Source: CAD feature listing. Evaluate the final solid. Frame: model axes, mm. A direction names the side the tool comes from. Give positions to 0.01 mm unless a question says otherwise; leave off trailing zeros. Loops run counter-clockwise (first coordinate to the right, second up) from the corner with the lowest first, then second, coordinate; pieces in that order, holes last. Notation, with made-up numbers: M 7.25,69.5 L 46.25,69.5 A34 ccw 46.25,99.5 Z; hole C 59,-11 d3. An arc over 180 degrees is marked long. Put each result on its own line as item: value. Start each with the question number.
```python
from build123d import *

# Parameters (mm, degrees)
TOP_DEPTH          = 30
PROFILE_3_W        = 96
PROFILE_3_H        = 17
SIDE_DEPTH         = 3
PROFILE_6_W        = 96
PROFILE_6_H        = 3
BEND_DEPTH         = 9
SCREWPLATE_START   = -7
PROFILE_7_R        = 2.5
PROFILE_7_R_2      = 2
SCREWPLATE_DEPTH   = 2
SIDE2_START        = -30
PROFILE_8_W        = 96
PROFILE_8_H        = 17
SIDE2_DEPTH        = 3
BEND2_START        = -30
PROFILE_9_W        = 96
PROFILE_9_H        = 3
BEND2_DEPTH        = 9
SCREWPLATE2_START  = -21
PROFILE_10_R       = 2.5
PROFILE_10_R_2     = 2
SCREWPLATE2_DEPTH  = 2
SKETCH3_R          = 2
CUT_EXTRUDE4_DEPTH = 2
CUT_EXTRUDE5_START = -1
SKETCH3_3_R        = 4
SKETCH3_3_R_2      = 2
CUT_EXTRUDE5_DEPTH = 1


with BuildPart() as part:
    # Profile → Top (new body)
    with BuildSketch(Plane.XY):
        Polygon((97.259067876, 0), (87.259067876, 0), (-32.740932124, 0), (-42.740932124, 0), (-42.740932124, 2), (97.259067876, 2), align=None)
    extrude(amount=-TOP_DEPTH)

    # Profile<3> → Side (add)
    with BuildSketch(Plane.XY):
        with Locations((27.259067876, -8.5)):
            Rectangle(PROFILE_3_W, PROFILE_3_H)
    extrude(amount=-SIDE_DEPTH)

    # Profile<6> → Bend (add)
    with BuildSketch(Plane.XY):
        with Locations((27.259067876, -18.5)):
            Rectangle(PROFILE_6_W, PROFILE_6_H)
    extrude(amount=-BEND_DEPTH)

    # Profile<7> → ScrewPlate (add)
    with BuildSketch(Plane.XY.offset(SCREWPLATE_START)):
        Polygon((75.259067876, -20), (-20.740932124, -20), (-20.740932124, -35), (7.259067876, -35), (7.259067876, -60), (27.259067876, -60), (47.259067876, -60), (47.259067876, -35), (75.259067876, -35), align=None)
        with Locations((17.259067876, -47.5)):
            Circle(PROFILE_7_R, mode=Mode.SUBTRACT)
        with Locations((37.259067876, -47.5)):
            Circle(PROFILE_7_R, mode=Mode.SUBTRACT)
        with Locations((-15.740932124, -27)):
            Circle(PROFILE_7_R_2, mode=Mode.SUBTRACT)
        with Locations((70.259067876, -27)):
            Circle(PROFILE_7_R_2, mode=Mode.SUBTRACT)
    extrude(amount=-SCREWPLATE_DEPTH)

    # Profile<8> → Side2 (add)
    with BuildSketch(Plane.XY.offset(SIDE2_START)):
        with Locations((27.259067876, -8.5)):
            Rectangle(PROFILE_8_W, PROFILE_8_H)
    extrude(amount=SIDE2_DEPTH)

    # Profile<9> → Bend2 (add)
    with BuildSketch(Plane.XY.offset(BEND2_START)):
        with Locations((27.259067876, -18.5)):
            Rectangle(PROFILE_9_W, PROFILE_9_H)
    extrude(amount=BEND2_DEPTH)

    # Profile<10> → ScrewPlate2 (add)
    with BuildSketch(Plane.XY.offset(SCREWPLATE2_START)):
        Polygon((75.259067876, -20), (-20.740932124, -20), (-20.740932124, -35), (7.259067876, -35), (7.259067876, -60), (27.259067876, -60), (47.259067876, -60), (47.259067876, -35), (75.259067876, -35), align=None)
        with Locations((17.259067876, -47.5)):
            Circle(PROFILE_10_R, mode=Mode.SUBTRACT)
        with Locations((37.259067876, -47.5)):
            Circle(PROFILE_10_R, mode=Mode.SUBTRACT)
        with Locations((-15.740932124, -27)):
            Circle(PROFILE_10_R_2, mode=Mode.SUBTRACT)
        with Locations((70.259067876, -27)):
            Circle(PROFILE_10_R_2, mode=Mode.SUBTRACT)
    extrude(amount=-SCREWPLATE2_DEPTH)

    # Sketch3 → Cut-Extrude4 (cut)
    with BuildSketch(Plane(origin=(0, 2, 0), x_dir=(1, 0, 0), z_dir=(0, 1, 0))):
        with Locations(Location((19.259067876, 20, 0), (0, 0, 270))):
            Circle(SKETCH3_R)
        with Locations(Location((35.259067876, 20, 0), (0, 0, 270))):
            Circle(SKETCH3_R)
        with Locations(Location((35.259067876, 10, 0), (0, 0, 270))):
            Circle(SKETCH3_R)
        with Locations(Location((19.259067876, 10, 0), (0, 0, 270))):
            Circle(SKETCH3_R)
    extrude(amount=-CUT_EXTRUDE4_DEPTH, mode=Mode.SUBTRACT)

    # Sketch3<3> → Cut-Extrude5 (cut)
    # profile 1 of 4: a face of its own
    with BuildSketch(Plane(origin=(0, 2, 0), x_dir=(1, 0, 0), z_dir=(0, 1, 0)).offset(CUT_EXTRUDE5_START)):
        with Locations(Location((19.259067876, 20, 0), (0, 0, 270))):
            Circle(SKETCH3_3_R)
        with Locations(Location((19.259067876, 20, 0), (0, 0, 270))):
            Circle(SKETCH3_3_R_2, mode=Mode.SUBTRACT)
    # profile 2 of 4: a face of its own
    with BuildSketch(Plane(origin=(0, 2, 0), x_dir=(1, 0, 0), z_dir=(0, 1, 0)).offset(CUT_EXTRUDE5_START)):
        with Locations(Location((35.259067876, 20, 0), (0, 0, 270))):
            Circle(SKETCH3_3_R)
        with Locations(Location((35.259067876, 20, 0), (0, 0, 270))):
            Circle(SKETCH3_3_R_2, mode=Mode.SUBTRACT)
    # profile 3 of 4: a face of its own
    with BuildSketch(Plane(origin=(0, 2, 0), x_dir=(1, 0, 0), z_dir=(0, 1, 0)).offset(CUT_EXTRUDE5_START)):
        with Locations(Location((35.259067876, 10, 0), (0, 0, 270))):
            Circle(SKETCH3_3_R)
        with Locations(Location((35.259067876, 10, 0), (0, 0, 270))):
            Circle(SKETCH3_3_R_2, mode=Mode.SUBTRACT)
    # profile 4 of 4: a face of its own
    with BuildSketch(Plane(origin=(0, 2, 0), x_dir=(1, 0, 0), z_dir=(0, 1, 0)).offset(CUT_EXTRUDE5_START)):
        with Locations(Location((19.259067876, 10, 0), (0, 0, 270))):
            Circle(SKETCH3_3_R)
        with Locations(Location((19.259067876, 10, 0), (0, 0, 270))):
            Circle(SKETCH3_3_R_2, mode=Mode.SUBTRACT)
    extrude(amount=-CUT_EXTRUDE5_DEPTH, mode=Mode.SUBTRACT)


solid = part.part
```
1. Ray query, line 1 (Z direction, x = -7, y = -3.5); line 2 (Z direction, x = 37, y = -35); line 3 (Y direction, x = -10.5, z = -21.75). Return the intervals inside material, ascending.
2. Section D-D, the plane z = -19.75. Output: boundary loops of the cut face in (x, y).
3. Section C-C, the plane x = 28.5. Output: boundary loops of the cut face in (y, z).
4. Pull-direction query (Y, two-part tool) for faces 1 (the face through (27, -20, -3)), 2 (the face through (34, 1, -12)), 3 (the face through (33.485, 1.507, -9.077)); classes: released by +Y, released by -Y, zero draft, split by the parting line, or undercut.
5. Set-up query: faces 4 (the face through (34, 1, -22)), 5 (the face through (21.242, 1.507, -20.26)), 6 (the face through (27, -17, -24)). Return all of +Z, -Z, +X, -X, +Y, -Y with unobstructed straight access to the full face (end or side cutting, diameter ignored); none if empty.
6. Section A-A, the plane y = -27. Output: boundary loops of the cut face in (x, z).
7. Contact query for flat-ended pins moving along their axis: pin 1 (4.5 mm diameter, centred on x = 70.26, y = -27, fed in from -Z); pin 2 (4.5 mm diameter, centred on x = 37.26, y = -47.5, fed in from -Z); pin 3 (2 mm diameter, centred on y = -43.5, z = -8, fed in from -X); pin 4 (3.5 mm diameter, centred on x = 35.26, z = -20, fed in from +Y). Output: stop coordinate, or through.
8. Section B-B, the plane y = -13.5. Output: boundary loops of the cut face in (x, z), plus the area to 3 significant figures.
Results found:
1. line 1: -30 to -27, -3 to 0
1. line 2: -23 to -21, -9 to -7
1. line 3: -35 to -17, 0 to 2
2. outline: M -42.74,0 L 15.27,0 L 15.27,1 L 17.27,1 L 17.27,2 L -42.74,2 Z; M 21.24,1 L 23.25,1 L 23.25,0 L 31.27,0 L 31.27,1 L 33.27,1 L 33.27,2 L 21.24,2 Z; M 37.24,1 L 39.25,1 L 39.25,0 L 97.26,0 L 97.26,2 L 37.24,2 Z
3. outline: M -60,-23 L -20,-23 L -20,-30 L 2,-30 L 2,0 L -20,0 L -20,-7 L -60,-7 L -60,-9 L -17,-9 L -17,-3 L 0,-3 L 0,-27 L -17,-27 L -17,-21 L -60,-21 Z
4. face 1: released by -Y
4. face 2: undercut
4. face 3: zero draft
5. face 4: none
5. face 5: +Y
5. face 6: +X, -X
6. outline: M -20.74,-23 L -17.74,-23 L -17.74,-21 L -20.74,-21 Z; M -20.74,-9 L -17.74,-9 L -17.74,-7 L -20.74,-7 Z; M -13.74,-23 L 68.26,-23 L 68.26,-21 L -13.74,-21 Z; M -13.74,-9 L 68.26,-9 L 68.26,-7 L -13.74,-7 Z; M 72.26,-23 L 75.26,-23 L 75.26,-21 L 72.26,-21 Z; M 72.26,-9 L 75.26,-9 L 75.26,-7 L 72.26,-7 Z
7. pin 1: z = -23
7. pin 2: through
7. pin 3: x = 7.26
7. pin 4: y = -17
8. outline: M -20.74,-30 L 75.26,-30 L 75.26,-27 L -20.74,-27 Z; M -20.74,-3 L 75.26,-3 L 75.26,0 L -20.74,0 Z
8. area: 576 mm²
